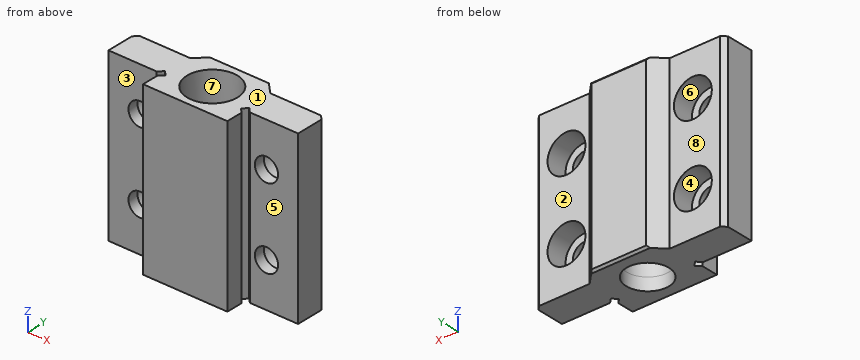
Autodesk Inventor part; units mm, degrees
ref_plane "YZ Plane" through (0, 0, 0) normal (1, 0, 0) x (0, 1, 0)
ref_plane "XZ Plane" through (0, 0, 0) normal (0, 1, 0) x (-1, 0, 0)
ref_plane "XY Plane" through (0, 0, 0) normal (0, 0, 1) x (1, 0, 0)
sketch "Sketch1" plane through (0, 0, 0) normal (0, 0, 1) x (1, 0, 0)
  line L0 (0, 0) -> (0, 31)
  line L1 (0, 0) -> (-20, 0)
  line L2 (-20, 0) -> (-20, 7.8787)
  line L3 (-22.1213, 10) -> (-45, 10)
  line L4 (-45, 10) -> (-45, 25)
  line L5 (-45, 25) -> (-19, 25)
  line L6 (-19, 25) -> (-13, 31)
  line L7 (-13, 31) -> (0, 31)
  line L8 (-22.1213, 10) -> (-20, 12.1213)
  line L9 (-20, 12.1213) -> (-17.8787, 10)
  line L10 (-17.8787, 10) -> (-20, 7.8787)
  line L11 (0, 0) -> (20, 0)
  line L12 (20, 0) -> (20, 7.8787)
  line L13 (22.1213, 10) -> (45, 10)
  line L14 (45, 10) -> (45, 25)
  line L15 (45, 25) -> (19, 25)
  line L16 (19, 25) -> (13, 31)
  line L17 (13, 31) -> (0, 31)
  line L18 (22.1213, 10) -> (20, 12.1213)
  line L19 (20, 12.1213) -> (17.8787, 10)
  line L20 (17.8787, 10) -> (20, 7.8787)
  dimension "d0" = 31
  dimension "d1" = 10
  dimension "d2" = 15
  dimension "d3" = 45
  dimension "d4" = 3
  dimension "d5" = 38
  dimension "d6" = 90
  dimension "d7" = 40
extrude "Extrusion1" add sketch "Sketch1" along normal mid plane 80
sketch "Sketch2" plane through (0, 0, 0) normal (1, 0, 0) x (0, 1, 0)
  line L0 (15, 40) -> (15, -40)
  line L1 (15, -40) -> (25.0727, -40)
  line L2 (25.0727, -40) -> (25.0727, -34)
  line L3 (25.0727, -34) -> (26.93, 40)
  line L4 (26.93, 40) -> (15, 40)
  line L5 (0, -40) -> (0, 40)
  point P0 (0, 0)
  point P1 (31, 40)
  point P2 (31, -40)
  dimension "d10" = 74
  dimension "d11" = 23.86
  dimension "d12" = 1.438
  dimension "d13" = 15
revolve "Revolution1" cut sketch "Sketch2" angle 360 about axis through (0, 15, 40) along (0, 0, -1)
sketch "Sketch3" plane through (19, 25, 40) normal (0, 1, 0) x (1, 0, 0)
  point P0 (-19, 40)
  point P1 (-49, 21)
  dimension "d15" = 19
  dimension "d16" = 30
hole "Hole1" at (-30, 25, 19) direction (0, -1, 0) diameter 11 end through all counterbore diameter 18 counterbore depth 10
pattern_linear "Rectangular Pattern1" count 2 spacing 60 along (1, 0, 0) count 2 spacing 38 along (0, 0, -1) of "Hole1"
chamfer "Chamfer1" distance 2 angle 45 2 edges at (-45, 25, 0) (45, 25, 0)
chamfer "Chamfer2" distance 1 angle 45 2 edges at (0, 31, 40) (0, 31, -40)
properties part number "Part040. Tool Holder" material "Steel, Alloy"
Part model, mm, in its own coordinate system. Face numbers are marked on the shaded views. A direction names the side the tool comes from. Give positions to 0.01 mm unless a question says otherwise; leave off trailing zeros. Write each loop counter-clockwise with the first axis right and the second up, starting at its lowest first coordinate (ties: lowest second). Pieces come first, ordered by that corner, then holes. Notation, with made-up numbers: (79, 62) -> (86, 62) arc R13 cw to (86, 70) -> close; hole circle Ø4 at (-29.75, -38). An arc over 180 degrees is marked (long way). Put each result on its own line as item: value. Start each with the question number.
Item 1: Cut at B-B (x = -30). List the corners of the cut face in (y, z), then the cut area to 3 significant figures.
Item 2: Cut at D-D (z = -29). List the corners of the cut face in (x, y), then the cut area to 3 significant figures.
Item 3: Pull direction Y, two halves, no side cores. Call the marked faces 5, 6, 7 and 8: pulls with the +Y half, pulls with the -Y half, needs draft (parallel to the pull), parting line crosses it, or undercut.
Item 4: Wall check: L1, parallel to Z at x = 30, y = 19; L2, parallel to Y at x = -3, z = -16; L3, parallel to X at y = 11, z = 19. Give the ranges that are in metal, low to high. Write a range as [from, to].
Item 5: Cut at A-A (x = 0). List the corners of the cut face in (y, z), then the cut area to 3 significant figures.
Item 6: Cut at C-C (y = 21). State how many separate pieces and enclosed holes the cut face has, then the cut area to 3 significant figures.
Item 7: Which spindle directions (+Z, -Z, +X, -X, +Y, -Y) get a long thin tool onto all of the face, cutting with end or side? Do the marked faces 1, 2, 3 and 4. Say none if no direction does.
Item 8: Pin check, flat tips, straight feed: pin 1 Ø23.5 at (x, z) = (-30, -19) entering from -Y; pin 2 Ø4 at (y, z) = (4, -19) entering from +X; pin 3 Ø23.5 at (x, z) = (30, -19) entering from +Y; pin 4 Ø20 at (x, z) = (27.5, -15) entering from +Y. Stop position of each tip, or through.
Answer list:
1. outline: (10, -40) -> (25, -40) -> (25, -28) -> (15, -28) -> (15, -24.5) -> (10, -24.5) -> close; (10, -13.5) -> (15, -13.5) -> (15, -10) -> (25, -10) -> (25, 10) -> (15, 10) -> (15, 13.5) -> (10, 13.5) -> close; (10, 24.5) -> (15, 24.5) -> (15, 28) -> (25, 28) -> (25, 40) -> (10, 40) -> close
1. area: 730 mm2
2. outline: (-45, 10) -> (-22.12, 10) -> (-20, 12.12) -> (-17.88, 10) -> (-20, 7.88) -> (-20, 0) -> (20, 0) -> (20, 7.88) -> (17.88, 10) -> (20, 12.12) -> (22.12, 10) -> (45, 10) -> (45, 23) -> (43, 25) -> (19, 25) -> (13, 31) -> (-13, 31) -> (-19, 25) -> (-43, 25) -> (-45, 23) -> close; hole circle Ø20.4 at (0, 15)
2. area: 1,600 mm2
3. face 5: pulls with the -Y half
3. face 6: needs draft
3. face 7: undercut
3. face 8: pulls with the +Y half
4. L1: z = [-40, -28], [-10, 10], [28, 40]
4. L2: y = [0, 4.91], [25.09, 31]
4. L3: x = [-45, -35.5], [-24.5, -21.12], [-18.88, -10.68], [10.68, 18.88], [21.12, 24.5], [35.5, 45]
5. outline: (0, -40) -> (4.93, -40) -> (4.93, -34) -> (3.07, 40) -> (0, 40) -> close; (25.07, -40) -> (30, -40) -> (31, -39) -> (31, 39) -> (30, 40) -> (26.93, 40) -> (25.07, -34) -> close
5. area: 730 mm2
6. separate pieces: 2
6. enclosed holes: 4
6. area: 4,720 mm2
7. face 1: +Z, +X, -X, +Y, -Y
7. face 2: +Z, -Z, +X, +Y
7. face 3: +Z, -Z, -X, -Y
7. face 4: +Y
8. pin 1: stops at y = 0
8. pin 2: stops at x = 20
8. pin 3: stops at y = 25.75
8. pin 4: stops at y = 26.5
